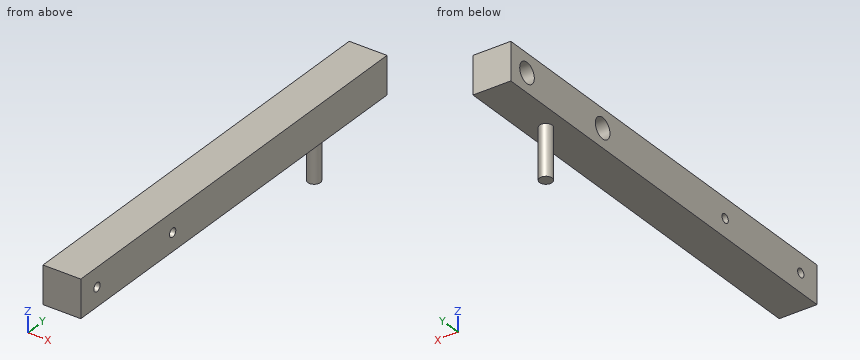
from build123d import *

# Parameters (mm, degrees)
SKETCH1_W           = 15
SKETCH1_H           = 15
BOSS_EXTRUDE1_DEPTH = 170
SKETCH2_R           = 1.75
CUT_EXTRUDE1_DEPTH  = 16
SKETCH3_R           = 4.05
CUT_EXTRUDE2_DEPTH  = 10
SKETCH5_R           = 2.5
BOSS_EXTRUDE3_DEPTH = 20


with BuildPart() as part:
    # Sketch1 → Boss-Extrude1 (new body)
    with BuildSketch(Plane(origin=(0, 0, 0), x_dir=(1, 0, 0), z_dir=(0, 1, 0))):
        Rectangle(SKETCH1_W, SKETCH1_H)
    extrude(amount=BOSS_EXTRUDE1_DEPTH)

    # Sketch2 → Cut-Extrude1 (cut, through all)
    with BuildSketch(Plane(origin=(7.5, 0, 0), x_dir=(0, 0, -1), z_dir=(1, 0, 0))):
        with Locations((0, 9)):
            Circle(SKETCH2_R)
        with Locations((0.295283966, 51)):
            Circle(SKETCH2_R)
    extrude(amount=-CUT_EXTRUDE1_DEPTH, mode=Mode.SUBTRACT)

    # Sketch3 → Cut-Extrude2 (cut)
    with BuildSketch(Plane.ZY.offset(7.5)):
        with Locations((0, 161)):
            Circle(SKETCH3_R)
        with Locations((0, 119)):
            Circle(SKETCH3_R)
    extrude(amount=-CUT_EXTRUDE2_DEPTH, mode=Mode.SUBTRACT)

    # Sketch5 → Boss-Extrude3 (add)
    with BuildSketch(Plane(origin=(0, 0, -7.5), x_dir=(-1, 0, 0), z_dir=(0, 0, -1))):
        with Locations((0, 140)):
            Circle(SKETCH5_R)
    extrude(amount=BOSS_EXTRUDE3_DEPTH)


solid = part.part
Can you work these out from the model? Positions are in its coordinate system, mm. Give positions to 0.01 mm unless a question says otherwise; leave off trailing zeros. Order: outer loops, then holes, each group sorted by start corner. A loop starts at its lowest first (then second) coordinate and runs counter-clockwise, first axis right, second up. Notation, with made-up numbers: M 56,55.25 L 91,55.25 A22 cw 91,79.25 Z; hole C 2.25,89 d7. An arc over 180 degrees is marked long. One line per item, written item: value.
Item 1: Please list where these lines run through material, in increasing order: line 1 (Y direction, x = -5.5, z = 0); line 2 (Y direction, x = 3.25, z = 0); line 3 (Z direction, x = -2, y = 62).
Verdict:
line 1: 0 to 7.25, 10.75 to 49.28, 52.72 to 114.95, 123.05 to 156.95, 165.05 to 170
line 2: 0 to 7.25, 10.75 to 49.28, 52.72 to 170
line 3: -7.5 to 7.5
Item 2: If we section it at D-D on z = 0: Write out the boundary of the cut face in (x, y), and give its area (3 significant figures).
Verdict:
outline: M -7.5,0 L 7.5,0 L 7.5,7.25 L -7.5,7.25 Z; M -7.5,10.75 L 7.5,10.75 L 7.5,49.28 L -7.5,49.28 Z; M -7.5,52.72 L 7.5,52.72 L 7.5,170 L -7.5,170 L -7.5,165.05 L 2.5,165.05 L 2.5,156.95 L -7.5,156.95 L -7.5,123.05 L 2.5,123.05 L 2.5,114.95 L -7.5,114.95 Z
area: 2,280 mm2
Item 3: If we section it at C-C on y = 140: Write out the boundary of the cut face in (x, z), and give its area (3 significant figures).
Verdict:
outline: M -7.5,-7.5 L -2.5,-7.5 L -2.5,-27.5 L 2.5,-27.5 L 2.5,-7.5 L 7.5,-7.5 L 7.5,7.5 L -7.5,7.5 Z
area: 325 mm2
Item 4: If we section it at A-A on y = 9: Write out the boundary of the cut face in (x, z).
Verdict:
outline: M -7.5,-7.5 L 7.5,-7.5 L 7.5,-1.75 L -7.5,-1.75 Z; M -7.5,1.75 L 7.5,1.75 L 7.5,7.5 L -7.5,7.5 Z
Item 5: If we section it at B-B on x = 0: Write out the boundary of the cut face in (y, z), and give its area (3 significant figures).
Verdict:
outline: M 0,-7.5 L 137.5,-7.5 L 137.5,-27.5 L 142.5,-27.5 L 142.5,-7.5 L 170,-7.5 L 170,7.5 L 0,7.5 Z; hole C 9,0 d3.5; hole C 51,-0.3 d3.5; hole C 119,0 d8.1; hole C 161,0 d8.1
area: 2,530 mm2
Item 6: For pin 1 (5 mm diameter, centred on y = 161, z = 0, fed in from -X); pin 2 (5 mm diameter, centred on x = 0, y = 78.5, fed in from -Z); pin 3 (3 mm diameter, centred on y = 137.5, z = -18, fed in from +X), each with a flat end and sliding along its axis, tell me the tip position at first contact or that it passes through.
Verdict:
pin 1: x = 2.5
pin 2: z = -7.5
pin 3: x = 2.29
